from build123d import *

# Parameters (mm, degrees)
BOSS_EXTRU_1_DEPTH      = 3.5
ESQUISSE2_R             = 2
ENL_V_MAT_EXTRU_1_DEPTH = 397.559259254
ESQUISSE3_R             = 1.5
ESQUISSE3_R_2           = 1.6
ENL_V_MAT_EXTRU_2_DEPTH = 397.559259254
ENL_V_MAT_EXTRU_3_DEPTH = 397.559259254


with BuildPart() as part:
    # Esquisse1 → Boss.-Extru.1 (new body)
    with BuildSketch(Plane.XY):
        with BuildLine():
            Line((5, 0), (245, 0))
            ThreePointArc((245, 0), (248.535533906, 1.464466094), (250, 5))
            Line((250, 5), (250, 302.81))
            ThreePointArc((250, 302.81), (248.535533906, 306.345533906), (245, 307.81))
            Line((245, 307.81), (5, 307.81))
            ThreePointArc((5, 307.81), (1.464466094, 306.345533906), (0, 302.81))
            Line((0, 302.81), (0, 5))
            ThreePointArc((0, 5), (1.464466094, 1.464466094), (5, 0))
        make_face()
    extrude(amount=BOSS_EXTRU_1_DEPTH)

    # Esquisse2 → Enlèv. mat.-Extru.1 (cut, through all)
    with BuildSketch(Plane.XY.offset(3.5)):
        with Locations((62, 8.5)):
            Circle(ESQUISSE2_R)
        with Locations((188, 8.5)):
            Circle(ESQUISSE2_R)
    extrude(amount=-ENL_V_MAT_EXTRU_1_DEPTH, mode=Mode.SUBTRACT)

    # Esquisse3 → Enlèv. mat.-Extru.2 (cut, through all)
    with BuildSketch(Plane.XY.offset(3.5)):
        with Locations((63, 155.81)):
            Circle(ESQUISSE3_R)
        with Locations((63, 282.81)):
            Circle(ESQUISSE3_R)
        with Locations((187, 282.81)):
            Circle(ESQUISSE3_R)
        with Locations((187, 155.81)):
            Circle(ESQUISSE3_R)
        with Locations((77.95, 243.58)):
            Circle(ESQUISSE3_R_2)
        with Locations((172.05, 243.58)):
            Circle(ESQUISSE3_R_2)
        with Locations((77.95, 195.04)):
            Circle(ESQUISSE3_R_2)
        with Locations((172.05, 195.04)):
            Circle(ESQUISSE3_R_2)
    extrude(amount=-ENL_V_MAT_EXTRU_2_DEPTH, mode=Mode.SUBTRACT)

    # Esquisse4 → Enlèv. mat.-Extru.3 (cut, through all)
    with BuildSketch(Plane.XY.offset(3.5)):
        with BuildLine():
            Line((90.28, 243.79), (159.72, 243.79))
            ThreePointArc((159.72, 243.79), (161.134213562, 243.204213562), (161.72, 241.79))
            Line((161.72, 241.79), (161.72, 196.83))
            ThreePointArc((161.72, 196.83), (161.134213562, 195.415786438), (159.72, 194.83))
            Line((159.72, 194.83), (90.28, 194.83))
            ThreePointArc((90.28, 194.83), (88.865786438, 195.415786438), (88.28, 196.83))
            Line((88.28, 196.83), (88.28, 241.79))
            ThreePointArc((88.28, 241.79), (88.865786438, 243.204213562), (90.28, 243.79))
        make_face()
    extrude(amount=-ENL_V_MAT_EXTRU_3_DEPTH, mode=Mode.SUBTRACT)


solid = part.part
Can you work these out from the model? Positions are in its coordinate system, mm. Give positions to 0.01 mm unless a question says otherwise; leave off trailing zeros. Answer as a JSON object with one key per item and string values. Group by question number.
Item 1: Suppose I cut it at A-A (z = 2.4). State how many separate pieces and enclosed holes the cut face has, plus the area to 3 significant figures.
Item 2: I'm going to push flat-ended pins straight in: P1, Ø3, axis at x = 159, y = 113, coming from the -Z side; P2, Ø1.9, axis at x = 172.05, y = 195.04, coming from the +Z side. Where does each tip first touch, or does it pass through?
Item 3: Please list where these lines run through material, in increasing order: line 1 (Y direction, x = 172.05, z = 1.4); line 2 (X direction, y = 155.81, z = 0.7); line 3 (X direction, y = 219, z = 0.9). Write a range as [from, to].
Findings:
{
 "1": {"separate pieces": "1", "enclosed holes": "11", "area": "73,300 mm²"},
 "2": {"P1": "stops at z = 0", "P2": "passes through"},
 "3": {"line 1": "y = [0, 193.44], [196.64, 241.98], [245.18, 307.81]", "line 2": "x = [0, 61.5], [64.5, 185.5], [188.5, 250]", "line 3": "x = [0, 88.28], [161.72, 250]"}
}
